Can you work these out from the model? Positions are in its coordinate system, mm. Face numbers are marked on the shaded views. A direction names the side the tool comes from. Round coordinates to 2 decimals unless told otherwise and drop trailing zeros. Loops run counter-clockwise (first coordinate to the right, second up) from the corner with the lowest first, then second, coordinate; pieces in that order, holes last.
from build123d import *

# Parameters (mm, degrees)
SKETCH_1_R          = 7.5
EXTRUDE_1_DEPTH     = 5
SKETCH_2_R          = 5
CUT_EXTRUDE_1_DEPTH = 2
SKETCH_3_R          = 3.4
CUT_EXTRUDE_2_DEPTH = 12.022703843
SKETCH_4_W          = 6
SKETCH_4_H          = 11
EXTRUDE_2_DEPTH     = 5


with BuildPart() as part:
    # 草图1 → 凸台-拉伸1 (new body)
    with BuildSketch(Plane(origin=(0, 0, 0), x_dir=(0, 0, -1), z_dir=(1, 0, 0))):
        Circle(SKETCH_1_R)
    extrude(amount=EXTRUDE_1_DEPTH)

    # 草图2 → 切除-拉伸1 (cut)
    with BuildSketch(Plane.ZY):
        Circle(SKETCH_2_R)
    extrude(amount=-CUT_EXTRUDE_1_DEPTH, mode=Mode.SUBTRACT)

    # 草图3 → 切除-拉伸2 (cut, through all)
    with BuildSketch(Plane.ZY.offset(-2)):
        Circle(SKETCH_3_R)
    extrude(amount=-CUT_EXTRUDE_2_DEPTH, mode=Mode.SUBTRACT)

    # 草图4 → 凸台-拉伸2 (add)
    with BuildSketch(Plane.ZY):
        with Locations((8, 0)):
            Rectangle(SKETCH_4_W, SKETCH_4_H)
        with Locations((-8, 0)):
            Rectangle(SKETCH_4_W, SKETCH_4_H)
    extrude(amount=-EXTRUDE_2_DEPTH)


solid = part.part
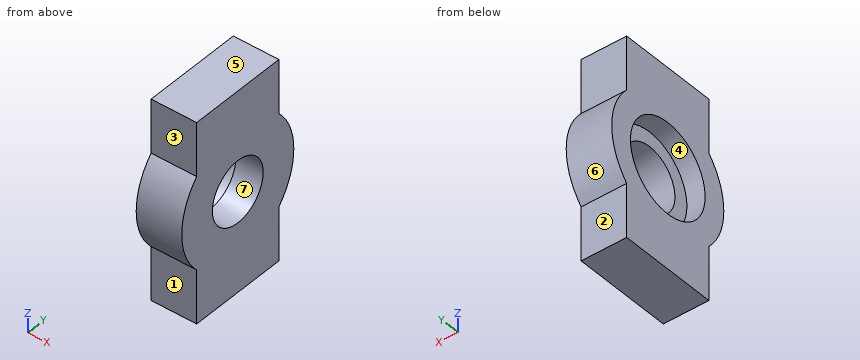
(1) Will these pins go through, and if not, where does the flat tip stop? P1, Ø1, axis at x = 2.5, z = -2.5, coming from the +Y side; P2, Ø2.5, axis at x = 2.5, z = -8, coming from the -Y side; P3, Ø5.5, axis at y = 0, z = 0, coming from the +X side; P4, Ø2.5, axis at x = 2.5, z = -8, coming from the +Y side.
Worked answers:
P1: stops at y = 7.23
P2: stops at y = -5.5
P3: passes through
P4: stops at y = 5.5
(2) For the marked faces 1, 2 and 3, which set-ups out of +Z, -Z, +X, -X, +Y, -Y let a thin tool reach every point of the face, with its end or its side?
Worked answers:
face 1: -Z, +X, -X, -Y
face 2: -Z, +X, -X, +Y
face 3: +Z, +X, -X, -Y
(3) If we section it at C-C, the plane z = 0: List the corners of the cut face in (x, y) for me, then the cut area to 3 significant figures.
Worked answers:
outline: (0, -7.5) - (5, -7.5) - (5, -3.4) - (2, -3.4) - (2, -5) - (0, -5) - close; (0, 5) - (2, 5) - (2, 3.4) - (5, 3.4) - (5, 7.5) - (0, 7.5) - close
area: 34.6 mm2
(4) If we section it at D-D, the plane x = 3.2: List the corners of the cut face in (y, z) for me, then the cut area to 3 significant figures.
Worked answers:
outline: (-5.5, -11) - (5.5, -11) - (5.5, -5.1) arc R7.5 ccw to (5.5, 5.1) - (5.5, 11) - (-5.5, 11) - (-5.5, 5.1) arc R7.5 ccw to (-5.5, -5.1) - close; hole circle Ø6.8 at (0, 0)
area: 234 mm2
(5) If we mould it in two halves opening along Y, with no side actions, what happens to the marked faces 4, 5, 6 and 7? For each: released by +Y, released by -Y, zero draft, split by the parting line, or undercut.
Worked answers:
face 4: undercut
face 5: zero draft
face 6: released by +Y
face 7: undercut
(6) If we section it at B-B, the plane y = 0: List the corners of the cut face in (x, z) for me.
Worked answers:
outline: (0, -11) - (5, -11) - (5, -3.4) - (2, -3.4) - (2, -5) - (0, -5) - close; (0, 5) - (2, 5) - (2, 3.4) - (5, 3.4) - (5, 11) - (0, 11) - close
(7) If we section it at A-A, the plane x = 1.35: List the corners of the cut face in (y, z) for me.
Worked answers:
outline: (-5.5, -11) - (5.5, -11) - (5.5, -5.1) arc R7.5 ccw to (5.5, 5.1) - (5.5, 11) - (-5.5, 11) - (-5.5, 5.1) arc R7.5 ccw to (-5.5, -5.1) - close; hole circle Ø10 at (0, 0)
(8) If I drill on line 1 (Z direction, x = 0.7, y = 0); line 2 (Y direction, x = 3.25, z = 8); line 3 (Y direction, x = 4.6, z = -2.75), over which ranges is the centre line in solid material (lowest first)?
Worked answers:
line 1: z = -11 to -5, 5 to 11
line 2: y = -5.5 to 5.5
line 3: y = -6.98 to -2, 2 to 6.98
